```python
from build123d import *

# Parameters (mm, degrees)
BASE_FLANGE1_DEPTH = 38.1
SKETCH6_R          = 2.413
CUT_EXTRUDE2_DEPTH = 2.54
SKETCH8_R          = 14.2875
CUT_EXTRUDE3_DEPTH = 2.54


# Sheet-metal steps are written as plain solids
with BuildPart() as part:
    # Sketch1 → Base-Flange1 (new body)
    with BuildSketch(Plane(origin=(0, 0, 0), x_dir=(0, 0, -1), z_dir=(1, 0, 0))):
        with BuildLine():
            Line((-25.4, 0), (-3.175, 0))
            ThreePointArc((-3.175, 0), (-0.92993597, -0.92993597), (0, -3.175))
            Line((0, -3.175), (0, -38.1))
            Line((0, -38.1), (-1.5875, -38.1))
            Line((-1.5875, -38.1), (-1.5875, -3.175))
            ThreePointArc((-1.5875, -3.175), (-2.052467985, -2.052467985), (-3.175, -1.5875))
            Line((-3.175, -1.5875), (-25.4, -1.5875))
            Line((-25.4, -1.5875), (-25.4, 0))
        make_face()
    extrude(amount=BASE_FLANGE1_DEPTH)

    # Sketch6 → Cut-Extrude2 (cut)
    with BuildSketch(Plane(origin=(0, 0, 0), x_dir=(1, 0, 0), z_dir=(0, 1, 0))):
        with Locations(Location((23.8125, -19.84375, 0), (0, 0, 270))):
            Circle(SKETCH6_R)
        with Locations(Location((19.05, -8.73125, 0), (0, 0, 270))):
            Circle(SKETCH6_R)
        with Locations(Location((14.2875, -19.84375, 0), (0, 0, 270))):
            Circle(SKETCH6_R)
    extrude(amount=-CUT_EXTRUDE2_DEPTH, mode=Mode.SUBTRACT)

    # Sketch8 → Cut-Extrude3 (cut)
    with BuildSketch(Plane(origin=(0, 0, 0), x_dir=(-1, 0, 0), z_dir=(0, 0, -1))):
        with Locations(Location((-19.05, -20.6375, 0), (0, 0, 90))):
            Circle(SKETCH8_R)
    extrude(amount=-CUT_EXTRUDE3_DEPTH, mode=Mode.SUBTRACT)


solid = part.part
```
Here's how the part is built. I have some questions about the finished solid (model axes, mm). A direction names the side the tool comes from. Round coordinates to 2 decimals unless told otherwise and drop trailing zeros. Write each loop counter-clockwise with the first axis right and the second up, starting at its lowest first coordinate (ties: lowest second). Pieces come first, ordered by that corner, then holes. Notation, with made-up numbers: M 28,1.5 L 49,1.5 A22 ccw 49,37.5 Z; hole C 54,7 d8. An arc over 180 degrees is marked long. Answer as CSV lines item,"result". Start each with the question number.
1. Suppose I cut it at B-B on z = 19.5. Write out the boundary of the cut face in (x, y), then the cut area to 3 significant figures.
2. On a 3-axis mill with a long thin cutter (end or side, diameter ignored), from which of +Z, -Z, +X, -X, +Y, -Y can I reach the whole of each face in a straight line? I mean faces 5 (the flat face through (10, -33, 1.588)), 6 (the cylindrical face through (21.442, -0.783, 8.417)). Say none if no direction works.
3. Suppose I cut it at C-C on y = -11.5. Write out the boundary of the cut face in (x, z), then the cut area to 3 significant figures.
4. Suppose I cut it at A-A on x = 19.05. Count the separate pieces of the cut face and the enclosed holes in it, then the cut area to 3 significant figures.
5. Thinking about a two-plate mould opening in Y: for faces 1 (the flat face through (19, -1.588, 14)), 2 (the cylindrical face through (18.78, -0.91, 0.95)), 3 (the flat face through (0, -13, 1)), 4 (the cylindrical face through (6.4, -14, 0.8)), which applies, released by +Y, released by -Y, zero draft, split by the parting line, or undercut?
6. I need wall thicknesses on probe 1 along Y at (x, z) = (16, 11); probe 2 along Z at (x, y) = (30, -9.5); probe 3 along Z at (x, y) = (36, -2). Which ranges of each line are inside material? Lowest first, please.
7. I'm going to push flat-ended pins straight in: pin 1 Ø5.5 at (x, z) = (23.81, 19.84) entering from -Y; pin 2 Ø10 at (x, z) = (26, 18.5) entering from +Y; pin 3 Ø3 at (x, z) = (26, 4) entering from -Y. Where does each tip first touch, or does it pass through?
Check result:
1,outline,"M 0,-1.59 L 11.9,-1.59 L 11.9,0 L 0,0 Z; M 16.68,-1.59 L 21.42,-1.59 L 21.42,0 L 16.68,0 Z; M 26.2,-1.59 L 38.1,-1.59 L 38.1,0 L 26.2,0 Z"
1,area,"45.3 mm2"
2,face 5,"+Z, +X, -X, -Y"
2,face 6,"+Y, -Y"
3,outline,"M 0,0 L 8.07,0 L 8.07,1.59 L 0,1.59 Z; M 30.03,0 L 38.1,0 L 38.1,1.59 L 30.03,1.59 Z"
3,area,"25.6 mm2"
4,separate pieces,"3"
4,enclosed holes,"0"
4,area,"43.6 mm2"
5,face 1,"released by -Y"
5,face 2,"released by +Y"
5,face 3,"zero draft"
5,face 4,"undercut"
6,probe 1,"y = -1.59 to 0"
6,probe 2,"z = 0 to 1.59"
6,probe 3,"z = 0.23 to 2.11"
7,pin 1,"stops at y = -1.59"
7,pin 2,"stops at y = 0"
7,pin 3,"stops at y = -1.74"
